from build123d import *


with BuildPart() as f1:
    # F0 (on Front) → F1 (revolve)
    with BuildSketch(Plane.XZ):
        with BuildLine():
            Line((75, 0), (75, 11.052214))
            ThreePointArc((75, 11.052214), (208.686368, 104.919376), (260, 260))
            Line((260, 260), (260, 710))
            ThreePointArc((260, 710), (208.686368, 865.080624), (75, 958.947786))
            Line((75, 958.947786), (75, 970))
            Line((75, 970), (50, 970))
            Line((50, 970), (50, 995))
            Line((50, 995), (0, 995))
            Line((0, 995), (0, 970))
            Line((0, 970), (0, 0))
            Line((0, 0), (0, -25))
            Line((0, -25), (50, -25))
            Line((50, -25), (50, 0))
            Line((50, 0), (75, 0))
        make_face()
    revolve(axis=Axis((0, 0, 485), (0, 0, -1)))


solid = f1.part
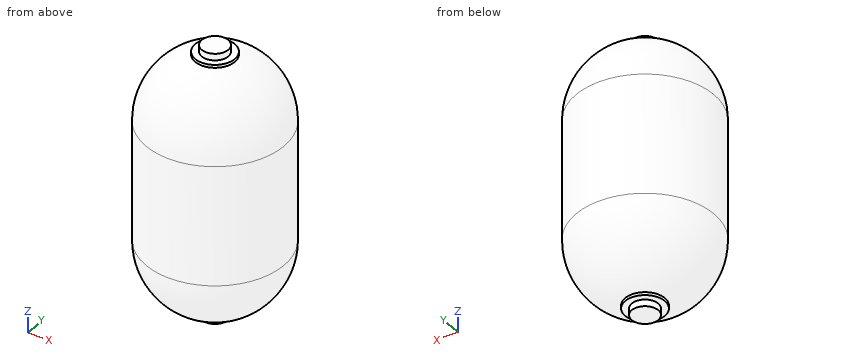
The listing builds one solid part. Answer for the finished solid, in the listing's coordinates (mm). Give positions to 0.01 mm unless a question says otherwise; leave off trailing zeros. Order: outer loops, then holes, each group sorted by start corner. A loop starts at its lowest first (then second) coordinate and runs counter-clockwise, first axis right, second up. Notation, with made-up numbers: (81.25, 15.5) - (124.25, 15.5) arc R33 ccw to (124.25, 43.5) - close; hole circle Ø6 at (49.25, -14). An arc over 180 degrees is marked (long way). Answer as CSV lines item,"result".
Q1. Each of these flat-tipped pins is pushed along its axis until it touches: pin 1 Ø1.5 at (x, z) = (-192, 146) entering from +Y; pin 2 Ø2 at (y, z) = (132, 132.5) entering from +X; pin 3 Ø4 at (x, z) = (173, 131.5) entering from +Y. Where does it stop, or does it pass through?
Answer key:
pin 1,"stops at y = 134.44"
pin 2,"stops at x = 185.16"
pin 3,"stops at y = 148.38"
Q2. Straight lines are drawn through the part: L1, parallel to X at y = 131, z = 361.5; L2, parallel to Y at x = -145, z = 196; L3, parallel to X at y = 13, z = 834.5. For each, find the intervals that lie inside material, in ascending order.
Answer key:
L1,"x = -224.59 to 224.59"
L2,"y = -206.1 to 206.1"
L3,"x = -227.88 to 227.88"
Q3. A cutting plane is placed at A-A, the plane z = 595. Determine the outline of the cut face in (x, y), and give its area (3 significant figures).
Answer key:
outline,"circle Ø520 at (0, 0)"
area,"212,000 mm^2"
